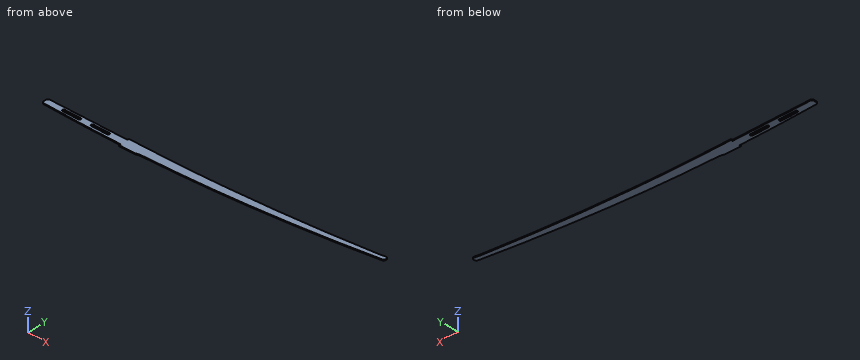
from build123d import *

# Parameters (mm, degrees)
EXTRUDE_1_DEPTH = 1.5


with BuildPart() as part:
    # 草图1 → 凸台-拉伸1 (new body, symmetric)
    with BuildSketch(Plane.XY):
        with BuildLine():
            Line((0, 12), (-244, 12))
            ThreePointArc((-244, 12), (-248.242640687, 10.242640687), (-250, 6))
            Line((-250, 6), (-250, -2.163248404))
            ThreePointArc((-250, -2.163248404), (-248.300744725, -6.346978177), (-244.165468396, -8.160966321))
            Line((-244.165468396, -8.160966321), (-170, -10.207084742))
            ThreePointArc((-170, -10.207084742), (-105.006181524, -11.551749873), (-40, -12))
            Line((-40, -12), (0, -12))
            Line((0, -12), (0, -17))
            Line((0, -17), (44.145576966, -17))
            ThreePointArc((44.145576966, -17), (49.047286744, -16.596845123), (53.817253308, -15.398216084))
            ThreePointArc((53.817253308, -15.398216084), (56.87159336, -14.535351182), (60, -14))
            ThreePointArc((60, -14), (69.983522822, -13.072941186), (80, -12.625335423))
            ThreePointArc((80, -12.625335423), (235.133064328, -6.904453143), (390, 3.82999502))
            ThreePointArc((390, 3.82999502), (578.273151109, 23.21141529), (765.76796239, 49.059328612))
            ThreePointArc((765.76796239, 49.059328612), (768.797355129, 50.747294353), (770, 54))
            Line((770, 54), (770, 57.675354294))
            ThreePointArc((770, 57.675354294), (768.391164992, 61.349588908), (764.6, 62.659328612))
            ThreePointArc((764.6, 62.659328612), (760.284727379, 62.197558708), (756, 61.507688779))
            ThreePointArc((756, 61.507688779), (748.020565474, 60.142412099), (740, 59.044284039))
            ThreePointArc((740, 59.044284039), (520.334050184, 36.766259367), (300, 22.541414161))
            ThreePointArc((300, 22.541414161), (180.031982479, 18.385538128), (60, 17))
            Line((60, 17), (0, 17))
            Line((0, 17), (0, 12))
        make_face()
        with BuildLine():
            Line((-50, -3), (-100, -3))
            ThreePointArc((-100, -3), (-104, 1), (-100, 5))
            Line((-100, 5), (-50, 5))
            ThreePointArc((-50, 5), (-46, 1), (-50, -3))
        make_face(mode=Mode.SUBTRACT)
        with BuildLine():
            Line((-140, -3), (-190, -3))
            ThreePointArc((-190, -3), (-194, 1), (-190, 5))
            Line((-190, 5), (-140, 5))
            ThreePointArc((-140, 5), (-136, 1), (-140, -3))
        make_face(mode=Mode.SUBTRACT)
    extrude(amount=EXTRUDE_1_DEPTH, both=True)


solid = part.part
Read the model definition and answer for the solid it produces. Units are mm, in the model's axes. Coordinates: 2 decimals unless noted, no trailing zeros. Order: outer loops, then holes, each group sorted by start corner. A loop starts at its lowest first (then second) coordinate and runs counter-clockwise, first axis right, second up. Notation, with made-up numbers: (47.5, 80) -> (55.5, 80) arc R20 ccw to (55.5, 116) -> close; hole circle Ø9 at (81, 58). An arc over 180 degrees is marked (long way). Answer as a JSON object with one key per item and string values.
1) A cutting plane is placed at A-A, the plane z = 0.45. State how many separate pieces and enclosed holes the cut face has, plus the area to 3 significant figures.
Model answer:
{"separate pieces": "1", "enclosed holes": "2", "area": "22,700 mm²"}
2) Consider line 1 along Y through (x, z) = (-22, -1.4); line 2 along Y through (x, z) = (423, 0.3); line 3 along Y through (x, z) = (-86, 0.25). Determine where each line is inside the solid, lowest interval first. Write a range as from..to.
Model answer:
{"line 1": "y = -12..12", "line 2": "y = 6.75..29.48", "line 3": "y = -11.78..-3, 5..12"}
3) A cutting plane is placed at D-D, the plane x = 156. Determine the outline of the cut face in (y, z), plus the area to 3 significant figures.
Model answer:
{"outline": "(-10.45, -1.5) -> (17.89, -1.5) -> (17.89, 1.5) -> (-10.45, 1.5) -> close", "area": "85.0 mm²"}
4) Each of these flat-tipped pins is pushed along its axis until it touches: pin 1 (0.9 mm diameter, centred on x = -94.5, z = 0, fed in from +Y); pin 2 (1.5 mm diameter, centred on x = -29.5, z = 0.5, fed in from -Y); pin 3 (1.5 mm diameter, centred on x = 21, z = 0.5, fed in from +Y). Where does it stop, or does it pass through?
Model answer:
{"pin 1": "stops at y = 12", "pin 2": "stops at y = -12", "pin 3": "stops at y = 17"}
